Autodesk Inventor part; units mm, degrees
ref_plane "YZ Plane" through (0, 0, 0) normal (1, 0, 0) x (0, 1, 0)
ref_plane "XZ Plane" through (0, 0, 0) normal (0, 1, 0) x (-1, 0, 0)
ref_plane "XY Plane" through (0, 0, 0) normal (0, 0, 1) x (1, 0, 0)
sketch "Esboço1" plane through (0, 0, 0) normal (0, 1, 0) x (-1, 0, 0)
  line L0 (55, -0.35) -> (55, -10)
  line L1 (67, -0.35) -> (67, -10)
  line L2 (67, -10) -> (55, -10)
  arc A0 (60.65, 1.6525) -> (58.35, 1.6525) centre (59.5, 3) ccw
  line L3 (58.35, 0) -> (58.35, 1.6525)
  line L4 (60.65, 0) -> (60.65, 1.6525)
  line L5 (60.65, 0) -> (60.65, -0.35)
  line L6 (60.65, -0.35) -> (67, -0.35)
  line L7 (58.35, 0) -> (58.35, -0.35)
  line L8 (58.35, -0.35) -> (55, -0.35)
  point P0 (0, 0)
  point P1 (-4, 56.431)
  dimension "d5" = 3.543
  dimension "d8" = 0.35
extrude "Extrusão1" add sketch "Esboço1" along normal blind 3
sketch "Esboço2" plane through (0, 3, 0) normal (0, 1, 0) x (1, 0, 0)
  point P0 (0, 0)
sketch "Esboço3" plane through (-67, 0, -10) normal (-1, 0, 0) x (0, 0, 1)
  line L0 (9.65, 0) -> (9.65, 3)
  line L1 (9.65, 0) -> (9.65, 3)
  line L2 (9.65, 3) -> (0, 3)
  line L3 (9.65, 3) -> (0, 3)
  line L4 (0, 0) -> (0, 3)
  line L5 (0, 3) -> (0, 0)
  line L6 (0, 0) -> (9.65, 0)
  point P0 (10, 0)
extrude "Extrusão2" add sketch "Esboço3" along normal blind 3
sketch "Esboço4" plane through (0, 3, 0) normal (0, 1, 0) x (1, 0, 0)
  arc A0 (-60.65, -1.6525) -> (-58.35, -1.6525) centre (-59.5, -3) ccw
  line L0 (-58.35, 0.35) -> (-55, 0.35)
  line L1 (-55, 0.35) -> (-55, -4.7715)
  line L2 (-60.65, 0.35) -> (-70, 0.35)
  line L3 (-70, 0.35) -> (-70, -4.7715)
  line L4 (-70, -4.7715) -> (-55, -4.7715)
  line L5 (-70, 0.35) -> (-70, 3.35)
  line L6 (-70, 10) -> (-70, 0.35)
  line L7 (-70, 3.35) -> (-55, 3.35)
  line L8 (-55, 3.35) -> (-55, 0.35)
  point P0 (0, 0)
  dimension "d14" = 3
extrude "Extrusão3" add sketch "Esboço4" along normal blind 3
sketch "Esboço5" plane through (0, 3, 0) normal (0, 1, 0) x (1, 0, 0)
  line L0 (-70, 10) -> (-55, 10)
  line L1 (-70, 3.35) -> (-55, 3.35)
  line L2 (-55, 10) -> (-70, 10)
  line L3 (-70, 10) -> (-70, 3.35)
  line L4 (-70, 3.35) -> (-55, 3.35)
  line L5 (-55, 3.35) -> (-55, 10)
  point P0 (0, 0)
extrude "Extrusão4" add sketch "Esboço5" along normal blind 3
sketch "Esboço6" plane through (0, 0, 0) normal (0, -1, 0) x (1, 0, 0)
  line L0 (-70, -0.35) -> (-70, 4.7715)
  line L1 (-70, -0.35) -> (-65, -0.35)
  line L2 (-60.65, -0.35) -> (-70, -0.35)
  line L3 (-65, -0.35) -> (-65, -5.35)
  line L4 (-65, -5.35) -> (-70, -5.35)
  line L5 (-70, -10) -> (-70, -0.35)
  line L6 (-70, -0.35) -> (-70, -5.35)
  point P0 (0, 0)
  dimension "d19" = 5
  dimension "d20" = 5
extrude "Extrusão5" add sketch "Esboço6" along normal blind 3
chamfer "Chanfro1" distance 3 angle 45 1 edges at (-67.5, 0, -5.35)
properties part number "encaixe suporte controlador L"
Geometry check sheet. Reference: the model listing, model coordinates, mm. A direction names the side the tool comes from. Coordinates: 2 decimals unless noted, no trailing zeros. Order: outer loops, then holes, each group sorted by start corner. A loop starts at its lowest first (then second) coordinate and runs counter-clockwise, first axis right, second up. Notation, with made-up numbers: M 10,-3.5 L 23,-3.5 A14 cw 23,11.5 Z; hole C 64,50 d4. An arc over 180 degrees is marked long. Answer as a JSON object with one key per item and string values.
Q1. Cross-section at C-C on y = 1. Record the cut outline in (x, z).
Results are:
{"outline": "M -70,-10 L -55,-10 L -55,-0.35 L -58.35,-0.35 L -58.35,1.65 A1.77 ccw long -60.65,1.65 L -60.65,-0.35 L -70,-0.35 Z"}
Q2. Release check for a two-part mould opening along Z. For faces 1 (the flat face through (-58.35, 1, 1)), 2 (the flat face through (-63, 4, 4.772)), 3 (the flat face through (-67.46, -1.48, -6.87)), 4 (the flat face through (-65, -1, -3)) record: released by +Z, released by -Z, zero draft, split by the parting line, or undercut.
Results are:
{"face 1": "undercut", "face 2": "released by +Z", "face 3": "released by -Z", "face 4": "zero draft"}
Q3. Cross-section at D-D on x = -56.5. Record the cut outline in (y, z), and give its area (3 significant figures).
Results are:
{"outline": "M 0,-10 L 6,-10 L 6,4.77 L 3,4.77 L 3,-0.35 L 0,-0.35 Z", "area": "73.3 mm²"}
Q4. Cross-section at A-A on z = 0. Record the cut outline in (x, y), and give its area (3 significant figures).
Results are:
{"outline": "M -70,3 L -60.65,3 L -60.65,0 L -58.35,0 L -58.35,3 L -55,3 L -55,6 L -70,6 Z", "area": "51.9 mm²"}
Q5. Depth check by flat-ended pin: pin 1 Ø1.5 at (x, z) = (-66.5, 2) entering from -Y; pin 2 Ø1 at (x, y) = (-58.5, -2) entering from +Z; pin 3 Ø1.6 at (y, z) = (1, 0.5) entering from +X. Enter the tip coordinate at first touch or a pass-through.
Results are:
{"pin 1": "stops at y = 3", "pin 2": "passes through", "pin 3": "stops at x = -58.35"}
Q6. Scan lines: line 1 (X direction, y = -2.25, z = -3); line 2 (Z direction, x = -65.25, y = 2.5); line 3 (Y direction, x = -55.25, z = -9.5). Record each from-to range of solid material in increasing order.
Results are:
{"line 1": "x = -70 to -65", "line 2": "z = -10 to -0.35", "line 3": "y = 0 to 6"}
Q7. Tool access check on faces 5 (the flat face through (-57, 1, -0.35)), 6 (the cylindrical face through (-59.44, 1.48, 4.77)), 7 (the flat face through (-60.65, 1, 1)), 8 (the flat face through (-55, 3, -4)). Record the directions out of +Z, -Z, +X, -X, +Y, -Y that give a thin tool (end or side, any length) a straight path to the whole face; none if there is none.
Results are:
{"face 5": "+X, -Y", "face 6": "-Y", "face 7": "-X, -Y", "face 8": "+Z, -Z, +X, +Y, -Y"}
